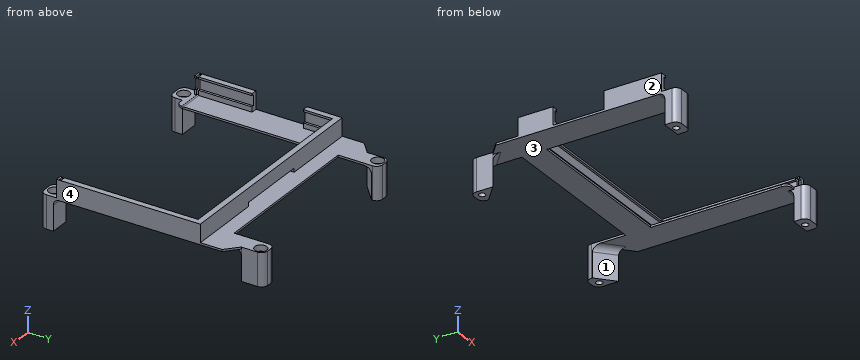
```python
from build123d import *

# Parameters (mm, degrees)
SKETCH1_W             = 6.535180092
SKETCH1_H             = 10
SKETCH1_R             = 1.6
BOSS_EXTRUDE1_DEPTH   = 15.5
BOSS_EXTRUDE1_2_DEPTH = 15.5
BOSS_EXTRUDE1_3_DEPTH = 15.5
BOSS_EXTRUDE1_4_DEPTH = 15.5
SKETCH2_R             = 1.6
BOSS_EXTRUDE2_DEPTH   = 1
SKETCH3_W             = 2.95
SKETCH3_H             = 28.672472045
BOSS_EXTRUDE3_DEPTH   = 2.5
BOSS_EXTRUDE4_DEPTH   = 5.4
SKETCH5_W             = 2.95
SKETCH5_H             = 28.672472045
BOSS_EXTRUDE5_DEPTH   = 1
SKETCH7_W             = 109
SKETCH7_H             = 1
CUT_EXTRUDE1_DEPTH    = 9
FILLET1_R             = 3
FILLET2_R             = 3
SKETCH8_W             = 35.6
SKETCH8_H             = 2
CUT_EXTRUDE2_DEPTH    = 2
SKETCH9_R             = 3
CUT_EXTRUDE3_DEPTH    = 3


with BuildPart() as part:
    # Sketch1 → Boss-Extrude1 (new body)
    with BuildSketch(Plane(origin=(0, 0, 0), x_dir=(0, 1, 0), z_dir=(0, 0, 1))):
        with Locations((-50.739127193, -49.754164457)):
            Rectangle(SKETCH1_W, SKETCH1_H)
        with Locations(Location((-50.006717239, -49.754164457, 0), (0, 0, 270))):
            Circle(SKETCH1_R, mode=Mode.SUBTRACT)
    extrude(amount=BOSS_EXTRUDE1_DEPTH)



with BuildPart() as body_2:
    # Sketch1 → Boss-Extrude1 2 (new body)
    with BuildSketch(Plane(origin=(0, 0, 0), x_dir=(0, 1, 0), z_dir=(0, 0, 1))):
        Polygon((42.477965747, -48.576148962), (50.136732851, -40.077363358), (53.691226628, -40.077363358), (53.691226628, -48.640781304), align=None)
        with Locations(Location((49.993282761, -45.101777457, 0), (0, 0, 270))):
            Circle(SKETCH1_R, mode=Mode.SUBTRACT)
    extrude(amount=BOSS_EXTRUDE1_2_DEPTH)


with BuildPart() as body_3:
    # Sketch1 → Boss-Extrude1 3 (new body)
    with BuildSketch(Plane(origin=(0, 0, 0), x_dir=(0, 1, 0), z_dir=(0, 0, 1))):
        Polygon((53.691226628, 49.132452389), (42.477965747, 49.067820047), (50.136732851, 40.569034443), (53.691226628, 40.569034443), align=None)
        with Locations(Location((49.993282761, 45.593448542, 0), (0, 0, 90))):
            Circle(SKETCH1_R, mode=Mode.SUBTRACT)
    extrude(amount=BOSS_EXTRUDE1_3_DEPTH)


with BuildPart() as body_4:
    # Sketch1 → Boss-Extrude1 4 (new body)
    with BuildSketch(Plane(origin=(0, 0, 0), x_dir=(0, 1, 0), z_dir=(0, 0, 1))):
        with Locations((-50.739127193, 50.245835543)):
            Rectangle(SKETCH1_W, SKETCH1_H)
        with Locations(Location((-50.006717239, 50.245835543, 0), (0, 0, 90))):
            Circle(SKETCH1_R, mode=Mode.SUBTRACT)
    extrude(amount=BOSS_EXTRUDE1_4_DEPTH)


with BuildPart() as part_1:
    add(part.part)

    add(body_2.part)  # Boss-Extrude2 merges body 2

    add(body_3.part)  # Boss-Extrude2 merges body 3

    add(body_4.part)  # Boss-Extrude2 merges body 4
    # Sketch2 → Boss-Extrude2 (add)
    with BuildSketch(Plane.XY.offset(15.5)):
        Polygon((54.754164457, -47.471537147), (54.754164457, -54.006717239), (44.754164457, -54.006717239), (44.754164457, -47.471537147), (40.077363358, -47.471537147), (40.077363358, 20.986771333), (-40.569034443, 20.986771333), (-40.569034443, -47.471537147), (-45.245835543, -47.471537147), (-45.245835543, -54.006717239), (-55.245835543, -54.006717239), (-55.245835543, -47.471537147), (-55.245835543, 36.910584236), (-49.067820047, 42.477965747), (-49.132452389, 53.691226628), (-40.569034443, 53.691226628), (-40.569034443, 33.42328432), (40.077363358, 33.42328432), (40.077363358, 53.691226628), (48.640781304, 53.691226628), (48.576148962, 42.477965747), (54.754164457, 36.910584236), align=None)
        with Locations((49.754164457, -50.006717239)):
            Circle(SKETCH2_R, mode=Mode.SUBTRACT)
        with Locations((45.101777457, 49.993282761)):
            Circle(SKETCH2_R, mode=Mode.SUBTRACT)
        with Locations(Location((-45.593448542, 49.993282761, 0), (0, 0, 180))):
            Circle(SKETCH2_R, mode=Mode.SUBTRACT)
        with Locations(Location((-50.245835543, -50.006717239, 0), (0, 0, 180))):
            Circle(SKETCH2_R, mode=Mode.SUBTRACT)
    extrude(amount=BOSS_EXTRUDE2_DEPTH)

    # Sketch3 → Boss-Extrude3 (add)
    with BuildSketch(Plane.XY.offset(16.5)):
        Polygon((-52.295835543, 8.439904174), (-52.295835543, 22.986771333), (51.804164457, 22.986771333), (51.804164457, -45.813228667), (54.754164457, -45.813228667), (54.754164457, 25.986771333), (-55.245835543, 25.986771333), (-55.245835543, 8.439904174), align=None)
        with Locations((-53.770835543, -31.476992645)):
            Rectangle(SKETCH3_W, SKETCH3_H)
    extrude(amount=BOSS_EXTRUDE3_DEPTH)

    # Sketch4 → Boss-Extrude4 (add)
    with BuildSketch(Plane.XY.offset(19)):
        Polygon((-55.245835543, 25.986771333), (54.754164457, 25.986771333), (54.754164457, -45.813228667), (52.954164457, -45.813228667), (52.954164457, -43.913228667), (52.954164457, 24.086771333), (-53.445835543, 24.086771333), (-53.445835543, 8.439904174), (-55.245835543, 8.439904174), align=None)
        Polygon((-55.245835543, -45.813228667), (-53.445835543, -45.813228667), (-53.445835543, -43.913228667), (-53.445835543, -17.140756622), (-55.245835543, -17.140756622), align=None)
    extrude(amount=BOSS_EXTRUDE4_DEPTH)

    # Sketch5 → Boss-Extrude5 (add)
    with BuildSketch(Plane.XY.offset(24.4)):
        Polygon((-55.245835543, 8.439904174), (-52.295835543, 8.439904174), (-52.295835543, 22.986771333), (51.804164457, 22.986771333), (51.804164457, -45.813228667), (54.754164457, -45.813228667), (54.754164457, 25.986771333), (-55.245835543, 25.986771333), align=None)
        with Locations((-53.770835543, -31.476992645)):
            Rectangle(SKETCH5_W, SKETCH5_H)
    extrude(amount=BOSS_EXTRUDE5_DEPTH)

    # Sketch7 → Cut-Extrude1 (cut)
    with BuildSketch(Plane.XY.offset(25.4)):
        with Locations((-0.245835543, -44.313228667)):
            Rectangle(SKETCH7_W, SKETCH7_H)
    extrude(amount=-CUT_EXTRUDE1_DEPTH, mode=Mode.SUBTRACT)

    # Fillet1
    fillet1_edges = [part_1.edges().sort_by_distance(p)[0] for p in [
        (48.640781304, 53.691226628, 7.75),
        (-49.132452389, 53.691226628, 7.75),
        (-40.569034443, -47.471537147, 16),
        (-55.245835543, -54.006717239, 8.25),
        (-45.245835543, -54.006717239, 8.25),
        (40.077363358, -47.471537147, 16),
        (44.754164457, -54.006717239, 8.25),
        (54.754164457, -54.006717239, 8.25),
        (40.077363358, 53.691226628, 7.75),
        (-40.569034443, 53.691226628, 7.75),
    ]]
    fillet(fillet1_edges, radius=FILLET1_R)

    # Fillet2
    # the kernel refuses this fillet: 3 mm, written as the material it adds along each edge
    with BuildSketch(Plane(origin=(54.147639825, 37.457160078, 15.5), x_dir=(0, 0, -1), z_dir=(-0.7428654483971854, 0.6694407558385198, 0))) as fillet2_piece_1_section:
        with BuildLine():
            CenterArc((FILLET2_R, FILLET2_R), FILLET2_R, 180, 90)
            Line((0, FILLET2_R), (0, 0))
            Line((0, 0), (FILLET2_R, 0))
        make_face()
    fillet2_piece_1 = extrude(amount=26.440545017, mode=Mode.PRIVATE)
    fillet2_piece_1 = split(fillet2_piece_1, bisect_by=Plane(origin=(48.592895704, 45.383408694, 14.829727011), z_dir=(-0.9999833890252455, 0.005763824562264406, 0)), keep=Keep.TOP, mode=Mode.PRIVATE)
    fillet2_piece_1 = split(fillet2_piece_1, bisect_by=Plane(origin=(40.077363358, 45.408013282, 14.829727011), z_dir=(1, 0, 0)), keep=Keep.TOP, mode=Mode.PRIVATE)
    add(fillet2_piece_1)
    with BuildSketch(Plane(origin=(-54.63931091, 37.457160078, 15.5), x_dir=(0, 0, -1), z_dir=(0.7428654483971854, 0.6694407558385198, 0))) as fillet2_piece_2_section:
        with BuildLine():
            CenterArc((FILLET2_R, -FILLET2_R), FILLET2_R, 90, 90)
            Line((0, -FILLET2_R), (0, 0))
            Line((0, 0), (FILLET2_R, 0))
        make_face()
    fillet2_piece_2 = extrude(amount=26.440545017, mode=Mode.PRIVATE)
    fillet2_piece_2 = split(fillet2_piece_2, bisect_by=Plane(origin=(-40.569034443, 45.408013282, 14.829727011), z_dir=(-1, 0, 0)), keep=Keep.TOP, mode=Mode.PRIVATE)
    fillet2_piece_2 = split(fillet2_piece_2, bisect_by=Plane(origin=(-49.084566789, 45.383408694, 14.829727011), z_dir=(0.9999833890252455, 0.005763824562264406, 0)), keep=Keep.TOP, mode=Mode.PRIVATE)
    add(fillet2_piece_2)
    with BuildSketch(Plane(origin=(-45.245835543, -47.471537147, 15.5), x_dir=(0, 0, -1), z_dir=(-1, 0, 0)), Plane(origin=(44.754164457, -47.471537147, 15.5), x_dir=(0, 1, 0), z_dir=(1, 0, 0))) as fillet2_piece_3:
        with BuildLine():
            CenterArc((FILLET2_R, -FILLET2_R), FILLET2_R, 90, 90)
            Line((0, -FILLET2_R), (0, 0))
            Line((0, 0), (FILLET2_R, 0))
        make_face()
    extrude(amount=10)

    # Sketch8 → Cut-Extrude2 (cut)
    with BuildSketch(Plane(origin=(0, 25.986771333, 0), x_dir=(-1, 0, 0), z_dir=(0, 1, 0))):
        with Locations((0.245835543, 17.5)):
            Rectangle(SKETCH8_W, SKETCH8_H)
    extrude(amount=-CUT_EXTRUDE2_DEPTH, mode=Mode.SUBTRACT)

    # Sketch9 → Cut-Extrude3 (cut)
    with BuildSketch(Plane.XY.offset(16.5)):
        with Locations((-45.593448542, 49.993282761)):
            Circle(SKETCH9_R)
        with Locations((-50.245835543, -50.006717239)):
            Circle(SKETCH9_R)
        with Locations(Location((49.754164457, -50.006717239, 0), (0, 0, 64.455545536))):
            Circle(SKETCH9_R)
        with Locations(Location((45.101777457, 49.993282761, 0), (0, 0, 180))):
            Circle(SKETCH9_R)
    extrude(amount=-CUT_EXTRUDE3_DEPTH, mode=Mode.SUBTRACT)


solid = part_1.part
```
Model file for the job. Use its own axes, mm. Face numbers are marked on the shaded views. A direction names the side the tool comes from. Coordinates: 2 decimals unless noted, no trailing zeros. Write each loop counter-clockwise with the first axis right and the second up, starting at its lowest first coordinate (ties: lowest second). Pieces come first, ordered by that corner, then holes. Notation, with made-up numbers: (-14, 53) - (25, 53) arc R19 ccw to (25, 68) - close; hole circle Ø8 at (33.25, -25). An arc over 180 degrees is marked (long way). Use a Markdown table: item, result. Add a question column.
Item 1: Band-saw the part on B-B, the plane y = -29.5. Write the cut outline in (x, z), and give its area (3 significant figures).
Item 2: 3-axis set-ups, long thin cutter, end or side, ignore diameter. For the marked faces 1 and 2: which of +Z, -Z, +X, -X, +Y, -Y reach the whole face in a straight line?
Item 3: Band-saw the part on D-D, the plane x = -1. Write the cut outline in (y, z), and give its area (3 significant figures).
Item 4: Drop flat-ended pins along their axis: pin 1 (4 mm diameter, centred on x = 20.5, z = 14, fed in from -Y); pin 2 (4.5 mm diameter, centred on x = 6.5, z = 22.5, fed in from -Y); pin 3 (12 mm diameter, centred on x = -39.5, z = 9, fed in from -Y); pin 4 (10 mm diameter, centred on y = 38, z = 13.5, fed in from -X). Give the stop position or say it passes through.
Item 5: Band-saw the part on A-A, the plane z = 3.5. Write the cut outline in (x, y), and give its area (3 significant figures).
Item 6: Band-saw the part on C-C, the plane z = 22.25. Write the cut outline in (x, y).
Item 7: Two-plate mould, pull along Y, no slides. Class the marked faces 3 and 4: pulls with the +Y half, pulls with the -Y half, needs draft (parallel to the pull), parting line crosses it, or undercut.
Item 8: Drill centre lines: line 1 along X through (y, z) = (25, 18); line 2 along X through (y, z) = (-35.5, 17); line 3 along Y through (x, z) = (-47, 13). Where is each one in solid material? Low to high.
A:
| question | item | result |
|---|---|---|
| 1 | outline | (-55.25, 15.5) - (-40.57, 15.5) - (-40.57, 16.5) - (-52.3, 16.5) - (-52.3, 19) - (-53.45, 19) - (-53.45, 24.4) - (-52.3, 24.4) - (-52.3, 25.4) - (-55.25, 25.4) - close; (40.08, 15.5) - (54.75, 15.5) - (54.75, 25.4) - (51.8, 25.4) - (51.8, 24.4) - (52.95, 24.4) - (52.95, 19) - (51.8, 19) - (51.8, 16.5) - (40.08, 16.5) - close |
| 1 | area | 69.4 mm² |
| 2 | face 1 | -Z |
| 2 | face 2 | +Z, -Z, -X, +Y, -Y |
| 3 | outline | (20.99, 15.5) - (33.42, 15.5) - (33.42, 16.5) - (23.99, 16.5) - (23.99, 18.5) - (25.99, 18.5) - (25.99, 25.4) - (22.99, 25.4) - (22.99, 24.4) - (24.09, 24.4) - (24.09, 19) - (22.99, 19) - (22.99, 16.5) - (20.99, 16.5) - close |
| 3 | area | 29.2 mm² |
| 4 | pin 1 | stops at y = 20.99 |
| 4 | pin 2 | stops at y = 22.99 |
| 4 | pin 3 | stops at y = -52.22 |
| 4 | pin 4 | stops at x = -55.25 |
| 5 | outline | (-55.25, -51.01) arc R3 ccw to (-52.25, -54.01) - (-48.25, -54.01) arc R3 ccw to (-45.25, -51.01) - (-45.25, -47.47) - (-55.25, -47.47) - close; (-49.12, 50.67) - (-49.07, 42.48) - (-40.57, 50.14) - (-40.57, 50.69) arc R3 ccw to (-43.57, 53.69) - (-46.12, 53.69) arc R3 ccw to start; (40.08, 50.14) - (48.58, 42.48) - (48.62, 50.67) arc R3 ccw to (45.62, 53.69) - (43.08, 53.69) arc R3 ccw to (40.08, 50.69) - close; (44.75, -51.01) arc R3 ccw to (47.75, -54.01) - (51.75, -54.01) arc R3 ccw to (54.75, -51.01) - (54.75, -47.47) - (44.75, -47.47) - close; hole circle Ø3.2 at (-50.25, -50.01); hole circle Ø3.2 at (-45.59, 49.99); hole circle Ø3.2 at (45.1, 49.99); hole circle Ø3.2 at (49.75, -50.01) |
| 5 | area | 209 mm² |
| 6 | outline | (-55.25, -45.81) - (-53.45, -45.81) - (-53.45, -44.81) - (-54.75, -44.81) - (-54.75, -43.81) - (-53.45, -43.81) - (-53.45, -17.14) - (-55.25, -17.14) - close; (-55.25, 8.44) - (-53.45, 8.44) - (-53.45, 24.09) - (52.95, 24.09) - (52.95, -43.81) - (54.25, -43.81) - (54.25, -44.81) - (52.95, -44.81) - (52.95, -45.81) - (54.75, -45.81) - (54.75, 25.99) - (-55.25, 25.99) - close |
| 7 | face 3 | undercut |
| 7 | face 4 | needs draft |
| 8 | line 1 | x = -55.25 to -18.05, 17.55 to 54.75 |
| 8 | line 2 | x = -55.25 to -52.3, 51.8 to 54.75 |
| 8 | line 3 | y = -53.74 to -47.43, 44.28 to 49.23, 50.76 to 53.56 |
